For this review, use the dimensioned drawing (mm, ordinates from the lowest corner) and the shaded views. A direction names the side the tool comes from. Give positions to 0.01 mm unless a question says otherwise; leave off trailing zeros. Loops run counter-clockwise (first coordinate to the right, second up) from the corner with the lowest first, then second, coordinate; pieces in that order, holes last. Notation, with made-up numbers: M 58,60.25 L 71,60.25 A5 ccw 71,69.25 Z; hole C 28,80.25 d10. An arc over 180 degrees is marked long. Use CSV: the item, a comma, the result in double quotes.
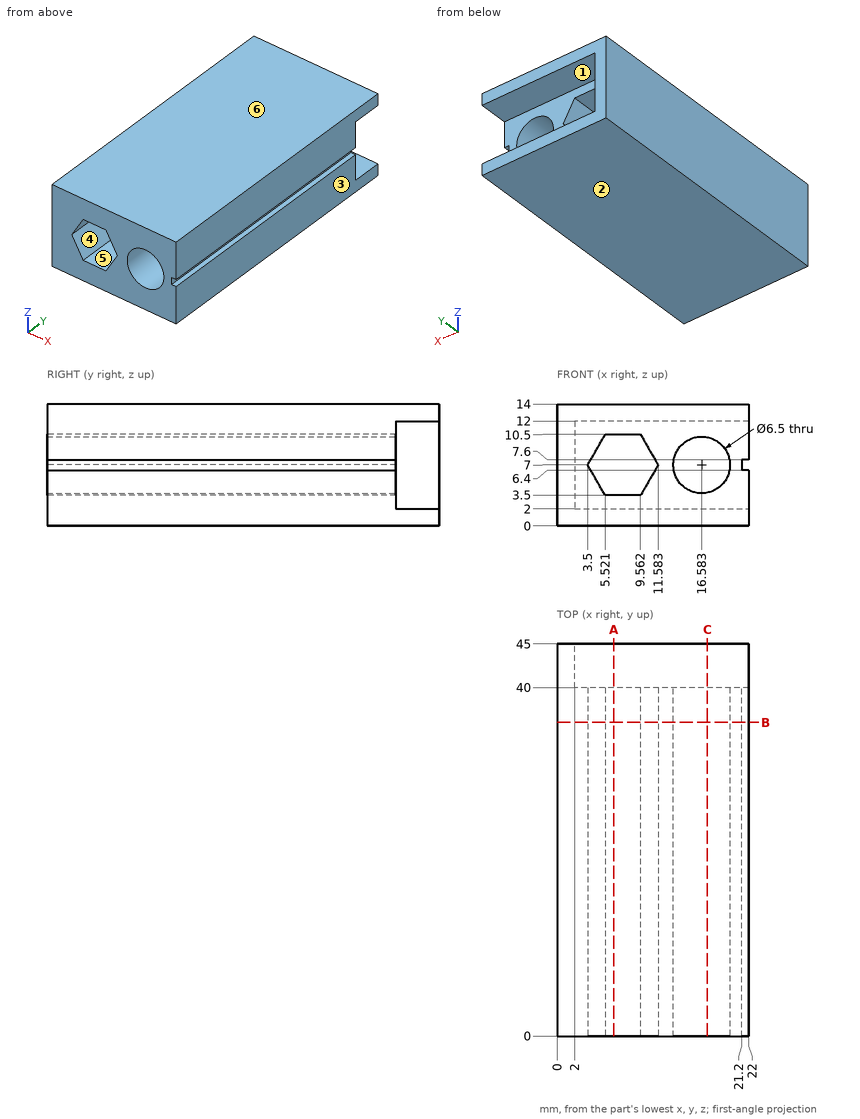
(1) We need section A-A on x = 6.5. State the section outline as (y, z) points, then the cut area to 3 significant figures.
A:
outline,"M 0,0 L 45,0 L 45,2 L 40,2 L 40,3.5 L 0,3.5 Z; M 0,10.5 L 40,10.5 L 40,12 L 45,12 L 45,14 L 0,14 Z"
area,"300 mm²"
(2) Machinability: for the marked faces 1 and 2, which of the approach directions +Z, -Z, +X, -X, +Y, -Y give a long, thin tool a straight path to every point of the face, cutting with its end or side? Answer none if there is none.
A:
face 1,"+X, +Y"
face 2,"-Z, +X, -X, +Y, -Y"
(3) Wall thickness on line 1 along X through (y, z) = (15.5, 7); line 2 along X through (y, z) = (26.5, 7.5) (1 decimal); line 3 along Z through (x, y) = (13.5, 43): over which ranges is each line inside the solid? List them lowest first. Write a range as [from, to].
A:
line 1,"[0, 3.5], [11.58, 13.33], [19.83, 21.2]"
line 2,"[0, 3.8], [11.3, 13.4], [19.8, 21.2]"
line 3,"[0, 2], [12, 14]"
(4) The part is to be moulded in two halves that separate along X. For the marked faces 3, 4, 5 and 6, say which applies: released by +X, released by -X, zero draft, split by the parting line, or undercut.
A:
face 3,"released by +X"
face 4,"undercut"
face 5,"undercut"
face 6,"zero draft"
(5) Clearance check with flat-ended pins moving along their axes: P1, Ø2.5, axis at y = 42, z = 9, coming from the +X side; P2, Ø3, axis at x = 15.5, z = 5, coming from the +Y side; P3, Ø0.6, axis at y = 10.5, z = 7, coming from the +X side. State where each tip first meets the part, or that it passes through.
A:
P1,"x = 2"
P2,"y = 40"
P3,"x = 21.2"
(6) We need section B-B on y = 36. State the section outline as (x, z) points, then the cut area to 3 significant figures.
A:
outline,"M 0,0 L 22,0 L 22,6.4 L 21.2,6.4 L 21.2,7.6 L 22,7.6 L 22,14 L 0,14 Z; hole M 3.5,7 L 5.52,3.5 L 9.56,3.5 L 11.58,7 L 9.56,10.5 L 5.52,10.5 Z; hole C 16.58,7 d6.5"
area,"231 mm²"
(7) We need section C-C on x = 17.25. State the section outline as (y, z) points.
A:
outline,"M 0,0 L 45,0 L 45,2 L 40,2 L 40,3.82 L 0,3.82 Z; M 0,10.18 L 40,10.18 L 40,12 L 45,12 L 45,14 L 0,14 Z"
